```python
from build123d import *

# Parameters (mm, degrees)
SKETCH1_W           = 132
SKETCH1_H           = 72
BOSS_EXTRUDE1_DEPTH = 2
SKETCH2_W           = 60
SKETCH2_H           = 3.570225369
BOSS_EXTRUDE2_DEPTH = 10


with BuildPart() as part:
    # Sketch1 → Boss-Extrude1 (new body)
    with BuildSketch(Plane.XY):
        Rectangle(SKETCH1_W, SKETCH1_H)
    extrude(amount=BOSS_EXTRUDE1_DEPTH)

    # Sketch2 → Boss-Extrude2 (add)
    with BuildSketch(Plane.XY.offset(2)):
        with Locations((11, 34.214887316)):
            Rectangle(SKETCH2_W, SKETCH2_H)
    boss_extrude2 = extrude(amount=BOSS_EXTRUDE2_DEPTH)

    # Mirror1: Boss-Extrude2 across plane
    add(boss_extrude2.mirror(Plane.ZX))


solid = part.part
```
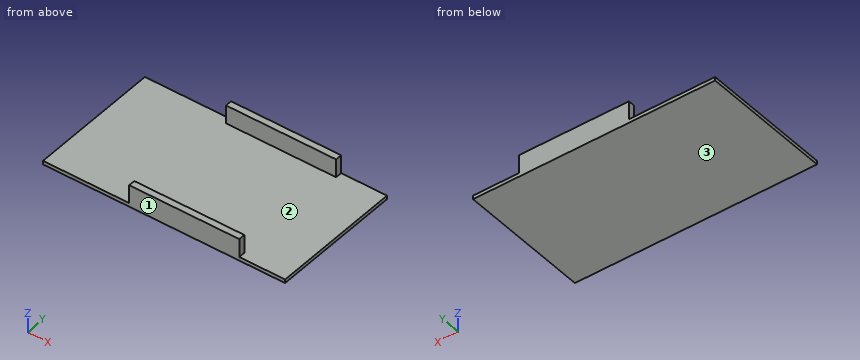
Geometry check sheet. Reference: the model listing, model coordinates, mm. Face numbers are marked on the shaded views. Round coordinates to 2 decimals unless told otherwise and drop trailing zeros. Loops run counter-clockwise (first coordinate to the right, second up) from the corner with the lowest first, then second, coordinate; pieces in that order, holes last. Notation, with made-up numbers: M -21,-21 L 3,-21 A32 ccw 3,13 Z; hole C 78.5,5.5 d9. An arc over 180 degrees is marked long. Return JSON: item names as keys, results as strings. Group by question number.
(1) Section check A-A, the plane z = 9. Enter the section's corners in (x, y).
(2) Section check B-B, the plane x = 25.5. Enter the section's corners in (y, z), and give its area (3 significant figures).
(3) Section check D-D, the plane x = -45. Enter the section's corners in (y, z).
(4) Mould release check, pull along Y, two halves, no side actions. Record for the marked faces 1, 2 and 3: pulls with the +Y half, pulls with the -Y half, needs draft (parallel to the pull), parting line crosses it, or undercut.
(5) Go/stop test with flat-tipped pins: pin 1 (1.8 mm diameter, centred on y = -34, z = 5.5, fed in from -X); pin 2 (4 mm diameter, centred on x = 24.5, y = 25, fed in from -Z); pin 3 (1.8 mm diameter, centred on y = 34.5, z = 7.5, fed in from +X); pin 4 (8 mm diameter, centred on x = -1.5, y = -18, fed in from +Z). Record where each tip stops, or that it passes through.
(6) Scan lines: line 1 along Y through (x, z) = (24, 3.75); line 2 along Z through (x, y) = (-27.5, -8.5). Record each from-to range of solid material in increasing order. Write a range as [from, to].
(7) Section check C-C, the plane y = -11. Enter the section's corners in (x, z), and give its area (3 significant figures).
Data:
{
 "1": {"outline": "M -19,-36 L 41,-36 L 41,-32.43 L -19,-32.43 Z; M -19,32.43 L 41,32.43 L 41,36 L -19,36 Z"},
 "2": {"outline": "M -36,0 L 36,0 L 36,12 L 32.43,12 L 32.43,2 L -32.43,2 L -32.43,12 L -36,12 Z", "area": "215 mm²"},
 "3": {"outline": "M -36,0 L 36,0 L 36,2 L -36,2 Z"},
 "4": {"face 1": "pulls with the -Y half", "face 2": "undercut", "face 3": "needs draft"},
 "5": {"pin 1": "x = -19", "pin 2": "z = 0", "pin 3": "x = 41", "pin 4": "z = 2"},
 "6": {"line 1": "[-36, -32.43], [32.43, 36]", "line 2": "[0, 2]"},
 "7": {"outline": "M -66,0 L 66,0 L 66,2 L -66,2 Z", "area": "264 mm²"}
}
